The model under review builds one solid part; all positions refer to its coordinate system, in mm. A direction names the side the tool comes from. Coordinates: 2 decimals unless noted, no trailing zeros. Write each loop counter-clockwise with the first axis right and the second up, starting at its lowest first coordinate (ties: lowest second). Pieces come first, ordered by that corner, then holes. Notation, with made-up numbers: (75.5, 16) - (96.5, 16) arc R29 ccw to (96.5, 36) - close; hole circle Ø10 at (15, 3.5). An arc over 180 degrees is marked (long way). Put each result on its own line as item: value.
from build123d import *

# Parameters (mm, degrees)
BOSS_EXTRUDE1_DEPTH = 45
CUT_EXTRUDE1_REACH  = 50.888
SKETCH2_R           = 1.274102828


with BuildPart() as part:
    # Sketch1 → Boss-Extrude1 (new body)
    with BuildSketch(Plane(origin=(0, 0, 0), x_dir=(1, 0, 0), z_dir=(0, 1, 0))):
        Polygon((-5, 13), (-14, 13), (-14, 0), (14, 0), (14, 13), (5, 13), (5, 5), (-5, 5), align=None)
    extrude(amount=BOSS_EXTRUDE1_DEPTH)

    # Sketch2 → Cut-Extrude1 (cut, up to next)
    with BuildSketch(Plane.XY, mode=Mode.PRIVATE) as cut_extrude1_sk1:
        with Locations((-10, 32.5)):
            Circle(SKETCH2_R)
    cut_extrude1_tool1 = extrude(cut_extrude1_sk1.sketch, amount=-CUT_EXTRUDE1_REACH, mode=Mode.PRIVATE) & part.part
    # Sketch2 → Cut-Extrude1 (cut, up to next)
    with BuildSketch(Plane.XY, mode=Mode.PRIVATE) as cut_extrude1_sk2:
        with Locations((10, 32.5)):
            Circle(SKETCH2_R)
    cut_extrude1_tool2 = extrude(cut_extrude1_sk2.sketch, amount=-CUT_EXTRUDE1_REACH, mode=Mode.PRIVATE) & part.part
    # Sketch2 → Cut-Extrude1 (cut, up to next)
    with BuildSketch(Plane.XY, mode=Mode.PRIVATE) as cut_extrude1_sk3:
        with Locations((10, 12.5)):
            Circle(SKETCH2_R)
    cut_extrude1_tool3 = extrude(cut_extrude1_sk3.sketch, amount=-CUT_EXTRUDE1_REACH, mode=Mode.PRIVATE) & part.part
    # Sketch2 → Cut-Extrude1 (cut, up to next)
    with BuildSketch(Plane.XY, mode=Mode.PRIVATE) as cut_extrude1_sk4:
        with Locations((-10, 12.5)):
            Circle(SKETCH2_R)
    cut_extrude1_tool4 = extrude(cut_extrude1_sk4.sketch, amount=-CUT_EXTRUDE1_REACH, mode=Mode.PRIVATE) & part.part
    add(cut_extrude1_tool1.solids().sort_by_distance((-10, 32.5, 0))[0], mode=Mode.SUBTRACT)
    add(cut_extrude1_tool2.solids().sort_by_distance((10, 32.5, 0))[0], mode=Mode.SUBTRACT)
    add(cut_extrude1_tool3.solids().sort_by_distance((10, 12.5, 0))[0], mode=Mode.SUBTRACT)
    add(cut_extrude1_tool4.solids().sort_by_distance((-10, 12.5, 0))[0], mode=Mode.SUBTRACT)


solid = part.part
1. Consider section A-A on z = -9.25. State the section outline as (x, y) points.
Determined:
outline: (-14, 0) - (-5, 0) - (-5, 45) - (-14, 45) - close; (5, 0) - (14, 0) - (14, 45) - (5, 45) - close; hole circle Ø2.55 at (-10, 12.5); hole circle Ø2.55 at (-10, 32.5); hole circle Ø2.55 at (10, 12.5); hole circle Ø2.55 at (10, 32.5)
2. Consider section D-D on z = -1.75. State the section outline as (x, y) points, plus the area to 3 significant figures.
Determined:
outline: (-14, 0) - (14, 0) - (14, 45) - (-14, 45) - close; hole circle Ø2.55 at (-10, 12.5); hole circle Ø2.55 at (-10, 32.5); hole circle Ø2.55 at (10, 12.5); hole circle Ø2.55 at (10, 32.5)
area: 1,240 mm^2
3. To check wall thickness, follow probe 1 along Y at (x, z) = (10, -4.25); probe 2 along X at (y, z) = (16.5, -6.5); probe 3 along Y at (x, z) = (-10.5, -10). State the ranges of each line that lie inside material, in increasing order.
Determined:
probe 1: y = 0 to 11.23, 13.77 to 31.23, 33.77 to 45
probe 2: x = -14 to -5, 5 to 14
probe 3: y = 0 to 11.33, 13.67 to 31.33, 33.67 to 45
4. Machinability: for faces 4 (the cylindrical face through (-11.273, 12.556, -6.409)), 5 (the flat face through (-5, 22, -9)), which of the approach directions +Z, -Z, +X, -X, +Y, -Y give a long, thin tool a straight path to every point of the face, cutting with its end or side? Answer none if there is none.
Determined:
face 4: +Z, -Z
face 5: -Z, +Y, -Y
5. Consider section C-C on x = 10. State the section outline as (y, z) points, plus the area to 3 significant figures.
Determined:
outline: (0, -13) - (11.23, -13) - (11.23, 0) - (0, 0) - close; (13.77, -13) - (31.23, -13) - (31.23, 0) - (13.77, 0) - close; (33.77, -13) - (45, -13) - (45, 0) - (33.77, 0) - close
area: 519 mm^2
6. The part is to be moulded in two halves that separate along Y. For faces 1 (the cylindrical face through (-10.276, 31.256, -6.409)), 2 (the flat face through (0, 0, -4)), 3 (the flat face through (0, 22, 0)), say which applies: +Y half, -Y half, draft (parallel to the pull), parting line (faces both ways), or undercut.
Determined:
face 1: undercut
face 2: -Y half
face 3: draft
7. Consider section B-B on y = 32.5. State the section outline as (x, z) points, plus the area to 3 significant figures.
Determined:
outline: (-14, -13) - (-11.27, -13) - (-11.27, 0) - (-14, 0) - close; (-8.73, -13) - (-5, -13) - (-5, -5) - (5, -5) - (5, -13) - (8.73, -13) - (8.73, 0) - (-8.73, 0) - close; (11.27, -13) - (14, -13) - (14, 0) - (11.27, 0) - close
area: 218 mm^2
8. For pin 1 Ø5 at (x, y) = (-0.5, 31) entering from -Z, flat-tipped, find the tip position at first contact; note if it passes through.
Determined:
pin 1: stops at z = -5
